The listing builds one solid part. Answer for the finished solid, in the listing's coordinates (mm). A direction names the side the tool comes from. Give positions to 0.01 mm unless a question says otherwise; leave off trailing zeros. Order: outer loops, then holes, each group sorted by start corner. A loop starts at its lowest first (then second) coordinate and runs counter-clockwise, first axis right, second up. Notation, with made-up numbers: (-7.5, 74.5) - (2.5, 74.5) arc R24 cw to (2.5, 98.5) - close; hole circle Ø8 at (-2.75, -19). An arc over 180 degrees is marked (long way). Use a Markdown table: item, result. Add a question column.
1) Find section B-B, the plane y = 15. Determine the outline of the cut face in (x, z), plus the area to 3 significant figures.
2) Find section D-D, the plane z = 10.25. Determine the outline of the cut face in (x, y), plus the area to 3 significant figures.
3) The mould has two halves that part along Z. Classify faces 1 (the face through (0, 9, -13)), 2 (the face through (0.105, 16.352, 8.974)), 3 (the face through (5, 4, 8)): released by +Z, released by -Z, zero draft, split by the parting line, or undercut.
4) Find section C-C, the plane x = -4.75. Determine the outline of the cut face in (y, z).
5) Find section A-A, the plane z = -7.5. Determine the outline of the cut face in (x, y).
6) Straight lines are drawn through the part: line 1 (Z direction, x = 4.5, y = 13.25); line 2 (Y direction, x = 0.5, z = -7.5); line 3 (Y direction, x = -4, z = -6). For each, find the intervals that lie inside material, in ascending order.
7) For faces 4 (the face through (2.5, 2, 9)), 5 (the face through (0, 9, 13)), determine the directions among +Z, -Z, +X, -X, +Y, -Y from which every point of the face is accessible in a straight line to the end or side of a thin tool.
8) A flat-ended cylindrical pin translates along its axis: pin 1 (2.5 mm diameter, centred on x = 4.5, z = 9, fed in from -Y). Find the tip coordinate at first contact, or state that the pin passes through.
Autodesk Inventor part; units mm, degrees
ref_plane "YZ Plane" through (0, 0, 0) normal (1, 0, 0) x (0, 1, 0)
ref_plane "XZ Plane" through (0, 0, 0) normal (0, 1, 0) x (-1, 0, 0)
ref_plane "XY Plane" through (0, 0, 0) normal (0, 0, 1) x (1, 0, 0)
sketch "Sketch1" plane through (0, 0, 0) normal (0, 1, 0) x (-1, 0, 0)
  line L0 (-7.5, 13) -> (7.5, 13)
  line L1 (7.5, 13) -> (7.5, -13)
  line L2 (7.5, -13) -> (-7.5, -13)
  line L3 (-7.5, -13) -> (-7.5, 13)
  line L4 (-7.5, 13) -> (7.5, -13) construction
  line L5 (7.5, 13) -> (-7.5, -13) construction
  point P0 (0, 0)
  dimension "d0" = 15
  dimension "d1" = 26
extrude "Extrusion1" add sketch "Sketch1" along normal blind 19
sketch "Sketch2" plane through (7.5, 0, 13) normal (1, 0, 0) x (0, 0, -1)
  line L0 (13, -3.8) -> (13, 22.8)
  circle A0 centre (5.5, 15) radius 2
  circle A1 centre (20.5, 15) radius 2
  line L1 (0, 0) -> (26, 0)
  point P0 (13, 0)
  dimension "d4" = 15
  dimension "d5" = 15
extrude "Extrusion2" cut sketch "Sketch2" against normal through all
sketch "Sketch3" plane through (7.5, 0, 13) normal (1, 0, 0) x (0, 0, -1)
  line L0 (26, 0) -> (0, 0)
  line L1 (0, 0) -> (9, 0)
  line L2 (9, 0) -> (9, 4)
  line L3 (9, 4) -> (0, 4)
  line L4 (0, 4) -> (0, 0)
  point P0 (13, 0)
  dimension "d8" = 4
  dimension "d9" = 9
extrude "Extrusion3" cut sketch "Sketch3" against normal blind 5
fillet "Fillet1" radius 2 7 edges at (0, 19, -13) (0, 19, 13) (0, 0, -13) (-2.5, 0, 13) (5, 4, 13) (5, 4, 4) (5, 0, 4)
properties part number "29_Lasercable_holder_A"
The answers:
| question | item | result |
|---|---|---|
| 1 | outline | (-7.5, -13) - (7.5, -13) - (7.5, -9.5) - (-7.5, -9.5) - close; (-7.5, -5.5) - (7.5, -5.5) - (7.5, 5.5) - (-7.5, 5.5) - close; (-7.5, 9.5) - (7.5, 9.5) - (7.5, 13) - (-7.5, 13) - close |
| 1 | area | 270 mm2 |
| 2 | outline | (-7.5, 0) - (2.5, 0) - (2.5, 4) - (7.5, 4) - (7.5, 19) - (-7.5, 19) - close |
| 2 | area | 265 mm2 |
| 3 | face 1 | released by -Z |
| 3 | face 2 | undercut |
| 3 | face 3 | zero draft |
| 4 | outline | (0, -11) arc R2 ccw to (2, -13) - (17, -13) arc R2 ccw to (19, -11) - (19, 11) arc R2 ccw to (17, 13) - (2, 13) arc R2 ccw to (0, 11) - close; hole circle Ø4 at (15, -7.5); hole circle Ø4 at (15, 7.5) |
| 5 | outline | (-7.5, 0) - (7.5, 0) - (7.5, 13) - (-7.5, 13) - close; (-7.5, 17) - (7.5, 17) - (7.5, 19) - (-7.5, 19) - close |
| 6 | line 1 | -13 to -8.47, -6.53 to 6.53, 8.47 to 13 |
| 6 | line 2 | 0 to 13, 17 to 19 |
| 6 | line 3 | 0 to 13.68, 16.32 to 19 |
| 7 | face 4 | +Z, +X, -Y |
| 7 | face 5 | +Z, +X, -X, +Y, -Y |
| 8 | pin 1 | y = 4 |
